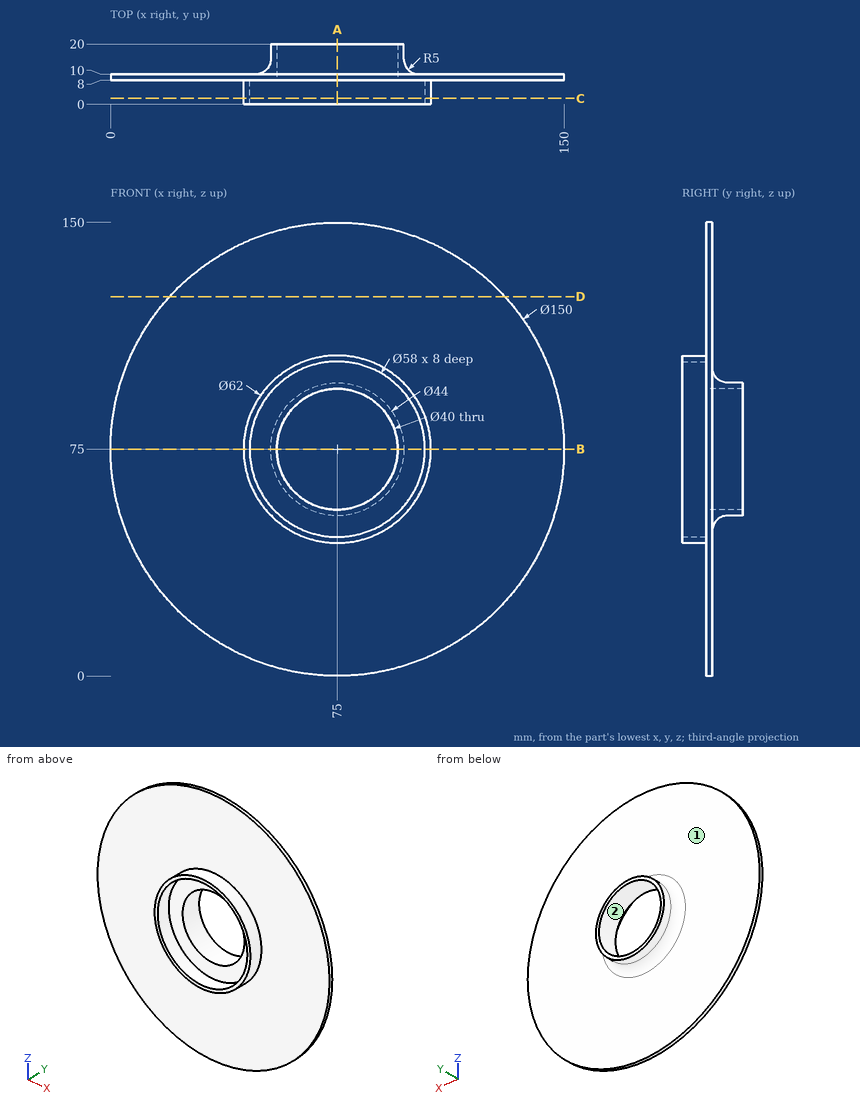
Can you work these out from the drawing? Everything is in mm from the part's minimum corner. Round coordinates to 2 decimals unless told otherwise and drop trailing zeros. Loops run counter-clockwise (first coordinate to the right, second up) from the corner with the lowest first, then second, coordinate; pieces in that order, holes last. Notation, with made-up numbers: (72.25, 59) - (119.25, 59) arc R24 cw to (119.25, 86) - close; hole circle Ø6 at (88, 88.25). An arc over 180 degrees is marked (long way). One line per question, with ' | ' between items. Start each with the question number.
Q1. Please list where these lines run through material, in increasing order: line 1 (Z direction, x = 75, y = 3.75); line 2 (Y direction, x = 53.5, z = 41.5); line 3 (Z direction, x = 75, y = 17.5). Write a range as [from, to].
Q2. I want a section at C-C (y = 2). Write out the boundary of the cut face in (x, z).
Q3. I want a section at B-B (z = 75). Write out the boundary of the cut face in (x, y), then the cut area to 3 significant figures.
Q4. I want a section at D-D (z = 125.5). Write out the boundary of the cut face in (x, y), then the cut area to 3 significant figures.
Q5. Will these pins go through, and if not, where does the flat tip stop? pin 1 (1.5 mm diameter, centred on x = 87, y = 8, fed in from +Z); pin 2 (3 mm diameter, centred on x = 21, y = 10.5, fed in from -Z); pin 3 (10 mm diameter, centred on y = 8.5, z = 29.5, fed in from -X).
Q6. I want a section at A-A (x = 75). Write out the boundary of the cut face in (y, z).
Q7. We'd pull the mould along X, two halves only. Please class the marked faces 1 and 2: +X half, -X half, draft (parallel to the pull), parting line (faces both ways), or undercut.
Response values:
1) line 1: z = [44, 46], [104, 106] | line 2: y = [8, 10] | line 3: z = [53, 55], [95, 97]
2) outline: circle Ø62 at (75, 75); hole circle Ø58 at (75, 75)
3) outline: (0, 8) - (44, 8) - (44, 0) - (46, 0) - (46, 8) - (55, 8) - (55, 20) - (53, 20) - (53, 15) arc R5 cw to (48, 10) - (0, 10) - close; (95, 8) - (104, 8) - (104, 0) - (106, 0) - (106, 8) - (150, 8) - (150, 10) - (102, 10) arc R5 cw to (97, 15) - (97, 20) - (95, 20) - close | area: 303 mm²
4) outline: (19.55, 8) - (130.45, 8) - (130.45, 10) - (19.55, 10) - close | area: 222 mm²
5) pin 1: stops at z = 149.15 | pin 2: stops at z = 21.52 | pin 3: stops at x = 11.88
6) outline: (0, 44) - (8, 44) - (8, 0) - (10, 0) - (10, 48) arc R5 cw to (15, 53) - (20, 53) - (20, 55) - (8, 55) - (8, 46) - (0, 46) - close; (0, 104) - (8, 104) - (8, 95) - (20, 95) - (20, 97) - (15, 97) arc R5 cw to (10, 102) - (10, 150) - (8, 150) - (8, 106) - (0, 106) - close
7) face 1: draft | face 2: undercut
